Autodesk Inventor part; units mm, degrees
ref_plane "YZ Plane" through (0, 0, 0) normal (1, 0, 0) x (0, 1, 0)
ref_plane "XZ Plane" through (0, 0, 0) normal (0, 1, 0) x (-1, 0, 0)
ref_plane "XY Plane" through (0, 0, 0) normal (0, 0, 1) x (1, 0, 0)
sketch "スケッチ1" plane through (0, 0, 0) normal (0, 1, 0) x (-1, 0, 0)
  line L0 (24, 0) -> (0, 0)
  line L1 (0, 0) -> (0, -26)
  line L2 (0, -26) -> (24, -26)
  line L3 (24, -26) -> (24, 0)
  circle A0 centre (24, -13) radius 13 construction
  circle A1 centre (24, -13) radius 12.5
  circle A2 centre (24, -13) radius 16
  point P0 (24, -25.5)
  point P1 (24, -0.5)
  point P2 (14.6726, 0)
  point P3 (14.6726, -26)
  dimension "d0" = 26
  dimension "d1" = 24
  dimension "d2" = 25
  dimension "d3" = 32
extrude "押し出し1" add sketch "スケッチ1" along normal blind 4 contours L3 A1 L2 A2 L0 | A2 L2 L1 L0 picked at (14.0879, -23.9339)
extrude "押し出し2" cut sketch "スケッチ1" along normal blind 2.2 contours L3 A1 L2 A2 L0 picked at (14.0879, -23.9339)
fillet "フィレット1" radius 1 4 edges at (-24, 3.1, -0.5) (-24, 3.1, 0) (-24, 3.1, -26) (-24, 3.1, -25.5)
sketch "スケッチ2" plane through (0, 4, 0) normal (0, 1, 0) x (1, 0, 0)
  circle A0 centre (-3, 2.5) radius 0.85 construction
  circle A1 centre (-3, 23.5) radius 0.85 construction
  circle A2 centre (-3, 2.5) radius 0.8
  circle A3 centre (-3, 23.5) radius 0.8
  point P0 (0, 0)
  dimension "d9" = 1.6
  dimension "d10" = 1.6
extrude "押し出し3" cut sketch "スケッチ2" against normal through all
sketch "スケッチ4" plane through (0, 4, 0) normal (0, 1, 0) x (1, 0, 0)
  line L0 (0, 26) -> (-17.8153, 26)
  line L1 (0, 0) -> (-1, 0)
  line L2 (-1, 0) -> (-1, 26)
  line L3 (-1, 26) -> (0, 26)
  line L4 (0, 26) -> (0, 0)
  dimension "d20" = 1
extrude "押し出し5" cut sketch "スケッチ4" against normal through all
sketch "スケッチ3" plane through (0, 4, 0) normal (0, 1, 0) x (1, 0, 0)
  circle A0 centre (-3, 2.5) radius 0.8
  circle A1 centre (-3, 23.5) radius 0.8
  circle A2 centre (-3, 2.5) radius 2
  circle A3 centre (-3, 23.5) radius 2
  point P0 (0, 0)
  dimension "d13" = 4
  dimension "d14" = 4
fillet "フィレット3" radius 2 3 edges at (-1, 4, -13) (-1, 2, 0) (-1, 2, -26)
extrude "押し出し6" cut sketch "スケッチ3" against normal blind 2
properties part number "joit_cover"
For this review, take the finished solid that the model builds, in its own axes (mm). A direction names the side the tool comes from. Coordinates: 2 decimals unless noted, no trailing zeros. Order: outer loops, then holes, each group sorted by start corner. A loop starts at its lowest first (then second) coordinate and runs counter-clockwise, first axis right, second up. Notation, with made-up numbers: (3, 87.5) - (30, 87.5) arc R13 cw to (30, 92.5) - close; hole circle Ø3 at (23, 68). An arc over 180 degrees is marked (long way). Answer as a JSON object with one key per item and string values. Group by question number.
1. For faces 4 (the flat face through (-11, 2.2, -13)), 5 (the flat face through (-6, 0, -13)), 6 (the flat face through (-2, 2, -3)), list the 3-axis set-ups (+Z, -Z, +X, -X, +Y, -Y) from which the entire face can be reached by the end or side of a thin tool; tool diameter is ignored.
2. We need section D-D on x = -9.25. State the section outline as (y, z) points, then the cut area to 3 significant figures.
3. We need section C-C on y = 2.5. State the section outline as (x, z) points, then the cut area to 3 significant figures.
4. We need section B-B on z = -22. State the section outline as (x, y) points.
5. Clearance check with flat-ended pins moving along their axes: P1, Ø3, axis at x = -3, z = -2.5, coming from the +Y side; P2, Ø3, axis at x = -13, z = -10.5, coming from the -Y side; P3, Ø1.3, axis at x = -3, z = -23.5, coming from the -Y side. State where each tip first meets the part, or that it passes through.
6. The part is to be moulded in two halves that separate along Z. For faces 1 (the cylindrical face through (-1.57, 3.4, -12.85)), 2 (the flat face through (-10, 2, -26)), 3 (the flat face through (-2, 2, -24)), say which applies: pulls with the +Z half, pulls with the -Z half, needs draft (parallel to the pull), parting line crosses it, or undercut.
7. For probe 1 along Z at (x, y) = (-3, 0.9); probe 2 along Z at (x, y) = (-3, 2.5); probe 3 along Z at (x, y) = (-12.25, 0.65), list the stretches that pass through material, from the lowest coordinate up.
8. We need section A-A on y = 1.1. State the section outline as (x, z) points, then the cut area to 3 significant figures.
Final values:
{
 "1": {"face 4": "-X, -Y", "face 5": "+Z, -Z, +X, -X, -Y", "face 6": "+Y"},
 "2": {"outline": "(0, -26) - (4, -26) - (4, 0) - (0, 0) - (0, -6.8) - (2.2, -6.8) - (2.2, -19.2) - (0, -19.2) - close", "area": "76.7 mm²"},
 "3": {"outline": "(-18.27, -24.11) arc R1 ccw to (-17.82, -26) - (-3, -26) arc R2 ccw to (-1.06, -24.5) - (-1.06, -24) arc R2 cw (long way) to (-1.06, -23) - (-1.06, -3) arc R2 cw (long way) to (-1.06, -2) - (-1.06, -1.5) arc R2 ccw to (-3, 0) - (-17.82, 0) arc R1 ccw to (-18.27, -1.89) arc R12.5 cw to start", "area": "315 mm²"},
 "4": {"outline": "(-15.33, 2.2) - (-10.77, 2.2) - (-10.77, 0) - (-1, 0) - (-1, 2) arc R2 ccw to (-1.68, 3.5) - (-1.68, 2) - (-4.32, 2) - (-4.32, 4) - (-15.33, 4) - close"},
 "5": {"P1": "y = 2", "P2": "y = 2.2", "P3": "through"},
 "6": {"face 1": "needs draft", "face 2": "pulls with the -Z half", "face 3": "undercut"},
 "7": {"probe 1": "-26 to -24.3, -22.7 to -3.3, -1.7 to 0", "probe 2": "-26 to -25.5, -21.5 to -4.5, -0.5 to 0", "probe 3": "-26 to -23.86, -2.14 to 0"},
 "8": {"outline": "(-14.67, -26) - (-3, -26) arc R2 ccw to (-1, -24) - (-1, -2) arc R2 ccw to (-3, 0) - (-14.67, 0) arc R16 cw to start; hole circle Ø1.6 at (-3, -23.5); hole circle Ø1.6 at (-3, -2.5)", "area": "228 mm²"}
}
